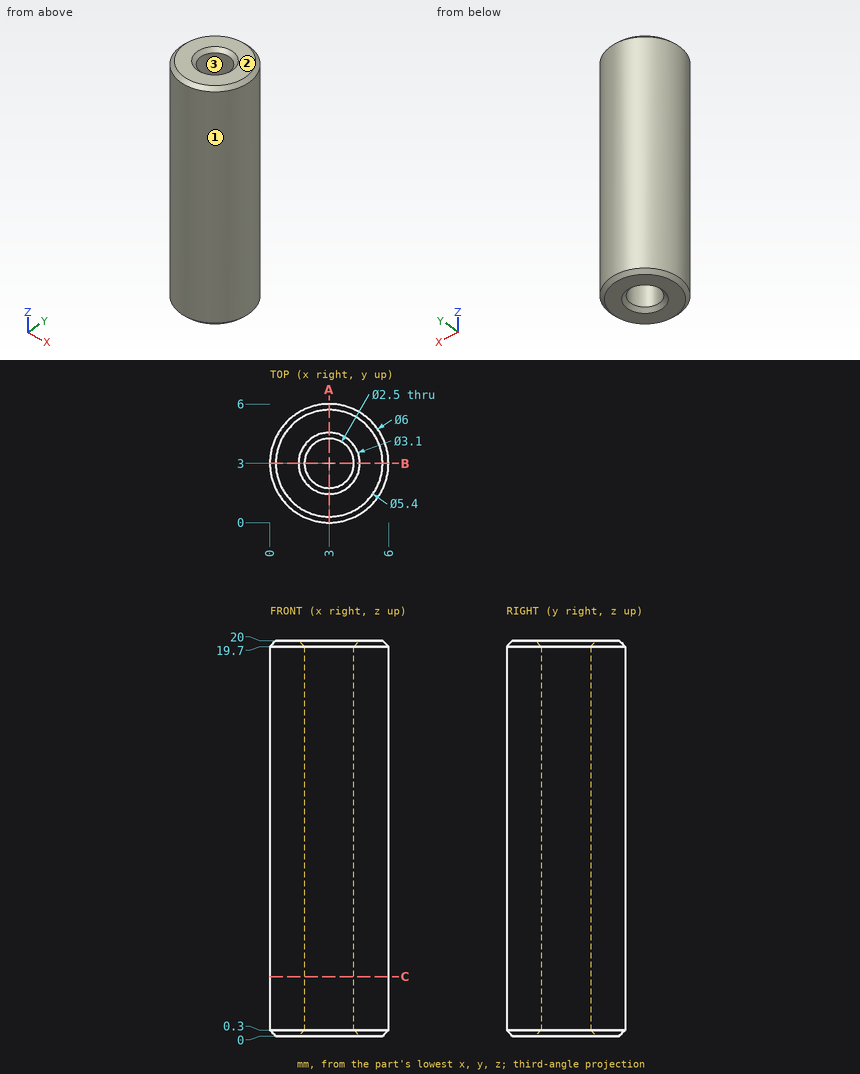
Design review of the part shown in the three views and the two pictorial views. Dimensions are in mm from the part's minimum x, y and z. Round coordinates to 2 decimals unless told otherwise and drop trailing zeros. Loops run counter-clockwise (first coordinate to the right, second up) from the corner with the lowest first, then second, coordinate; pieces in that order, holes last.
Q1. Mouldability with a two-part tool opening along Y and no side actions: class the marked faces 1, 2 and 3 as +Y half, -Y half, draft (parallel to the pull), parting line (faces both ways), or undercut.
Result sheet:
face 1: parting line
face 2: draft
face 3: undercut
Q2. Insertion check: pin 1 Ø1 at (x, z) = (5, 17.5) entering from -Y; pin 2 Ø1 at (y, z) = (4.5, 8) entering from -X. Each pin has a flat end and moves straight along its axis. Give the tip position at first contact, or say it passes through.
Result sheet:
pin 1: stops at y = 0.4
pin 2: stops at x = 0.17
Q3. Add section C-C on z = 3. Write out the cut boundary in (x, y), plus the area to 3 significant figures.
Result sheet:
outline: circle Ø6 at (3, 3); hole circle Ø2.5 at (3, 3)
area: 23.4 mm2
Q4. To check wall thickness, follow line 1 along Y through (x, z) = (3, 10); line 2 along Y through (x, z) = (2.35, 7.25); line 3 along X through (y, z) = (2.4, 7.25). State the ranges of each line that lie inside material, in increasing order.
Result sheet:
line 1: y = 0 to 1.75, 4.25 to 6
line 2: y = 0.07 to 1.93, 4.07 to 5.93
line 3: x = 0.06 to 1.9, 4.1 to 5.94
Q5. Add section A-A on x = 3. Write out the cut boundary in (y, z).
Result sheet:
outline: (0, 0.3) - (0.3, 0) - (1.45, 0) - (1.75, 0.3) - (1.75, 19.7) - (1.45, 20) - (0.3, 20) - (0, 19.7) - close; (4.25, 0.3) - (4.55, 0) - (5.7, 0) - (6, 0.3) - (6, 19.7) - (5.7, 20) - (4.55, 20) - (4.25, 19.7) - close
